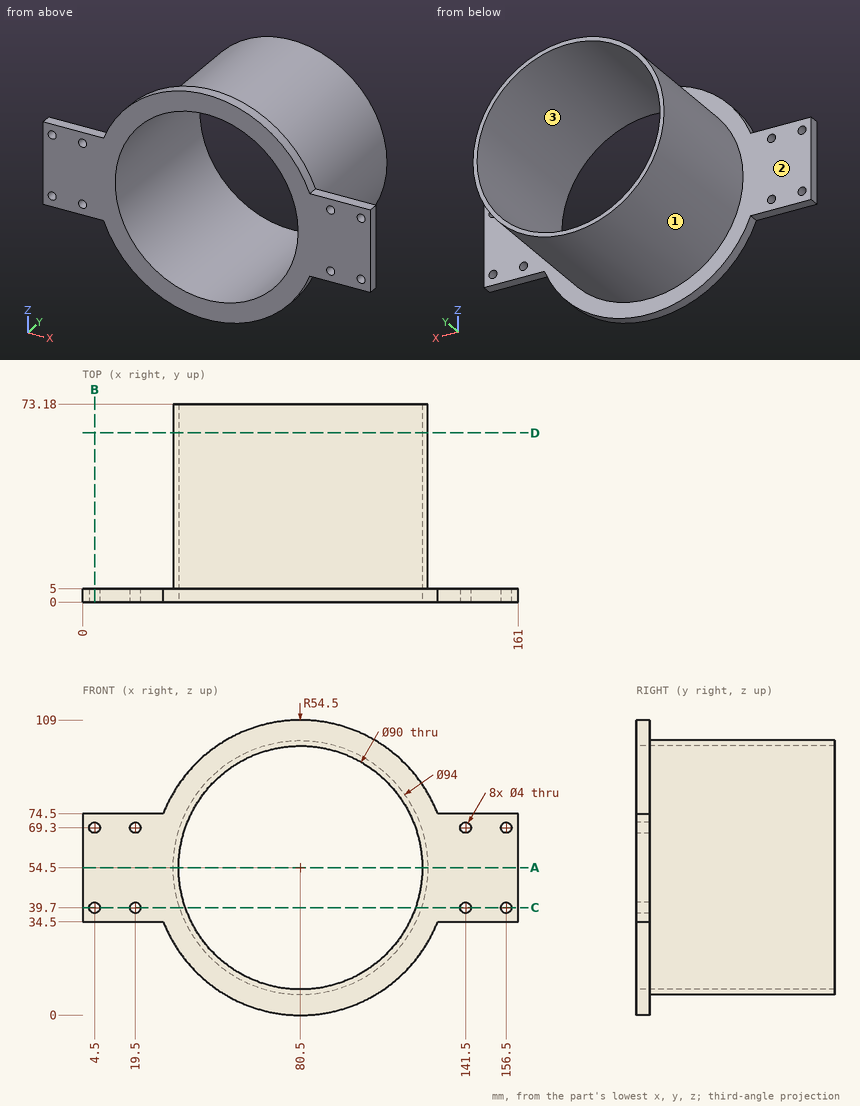
Could you check a few things on this drawing? It's one solid part, dimensions in mm from its lowest x, y, z. Give positions to 0.01 mm unless a question says otherwise; leave off trailing zeros. Write each loop counter-clockwise with the first axis right and the second up, starting at its lowest first coordinate (ties: lowest second). Pieces come first, ordered by that corner, then holes. Notation, with made-up numbers: M 77.25,50 L 113.25,50 A7 cw 113.25,55 Z; hole C 28,-3 d11. An arc over 180 degrees is marked long. Put each result on its own line as item: value. Start each with the question number.
Item 1: Thinking about a two-plate mould opening in X: for the marked faces 1, 2 and 3, which applies, +X half, -X half, draft (parallel to the pull), parting line (faces both ways), or undercut?
Item 2: If we section it at A-A, the plane z = 54.5: Write out the boundary of the cut face in (x, y).
Item 3: If we section it at B-B, the plane x = 4.5: Write out the boundary of the cut face in (y, z), then the cut area to 3 significant figures.
Item 4: If we section it at D-D, the plane y = 62.5: Write out the boundary of the cut face in (x, z), then the cut area to 3 significant figures.
Item 5: If we section it at C-C, the plane z = 39.7: Write out the boundary of the cut face in (x, y).
Item 6: I need wall thicknesses on L1, parallel to Z at x = 19.5, y = 1.9; L2, parallel to X at y = 2, z = 39; L3, parallel to X at y = 2.6, z = 39.7. Which ranges of each line are inside material? Lowest first, please. Write a range as from..to.
Item 7: Will these pins go through, and if not, where does the flat tip stop? pin 1 (4.5 mm diameter, centred on x = 19.5, z = 69.3, fed in from -Y); pin 2 (6 mm diameter, centred on x = 118.5, y = 25.5, fed in from +Z); pin 3 (5.5 mm diameter, centred on x = 7.5, y = 2, fed in from -Z); pin 4 (1.5 mm diameter, centred on x = 14, y = 3.5, fed in from +Z).
Values:
1. face 1: parting line
1. face 2: draft
1. face 3: undercut
2. outline: M 0,0 L 35.5,0 L 35.5,73.18 L 33.5,73.18 L 33.5,5 L 0,5 Z; M 125.5,0 L 161,0 L 161,5 L 127.5,5 L 127.5,73.18 L 125.5,73.18 Z
3. outline: M 0,34.5 L 5,34.5 L 5,37.7 L 0,37.7 Z; M 0,41.7 L 5,41.7 L 5,67.3 L 0,67.3 Z; M 0,71.3 L 5,71.3 L 5,74.5 L 0,74.5 Z
3. area: 160 mm²
4. outline: C 80.5,54.5 d94; hole C 80.5,54.5 d90
4. area: 578 mm²
5. outline: M 0,0 L 2.5,0 L 2.5,5 L 0,5 Z; M 6.5,0 L 17.5,0 L 17.5,5 L 6.5,5 Z; M 21.5,0 L 38,0 L 38,73.18 L 35.89,73.18 L 35.89,5 L 21.5,5 Z; M 123,0 L 139.5,0 L 139.5,5 L 125.11,5 L 125.11,73.18 L 123,73.18 Z; M 143.5,0 L 154.5,0 L 154.5,5 L 143.5,5 Z; M 158.5,0 L 161,0 L 161,5 L 158.5,5 Z
6. L1: 34.5..37.7, 41.7..67.3, 71.3..74.5
6. L2: 0..2.63, 6.37..17.63, 21.37..38.25, 122.75..139.63, 143.37..154.63, 158.37..161
6. L3: 0..2.5, 6.5..17.5, 21.5..38, 123..139.5, 143.5..154.5, 158.5..161
7. pin 1: y = 0
7. pin 2: z = 85.87
7. pin 3: z = 34.5
7. pin 4: z = 74.5
